Check sheet for the modelled part. Datum: model origin and axes. Units: mm. Face numbers are marked on the shaded views. A direction names the side the tool comes from. Coordinates: 2 decimals unless noted, no trailing zeros. Order: outer loops, then holes, each group sorted by start corner. A loop starts at its lowest first (then second) coordinate and runs counter-clockwise, first axis right, second up.
1. Set-up check for the marked faces 1 and 2: record each of +Z, -Z, +X, -X, +Y, -Y from which the full face is reachable in a straight line by a thin tool's end or side.
2. Cross-section at B-B (z = 38.1). Enter the section's corners in (x, y) (3 decimals).
3. Cross-section at D-D (x = -26). Enter the section's corners in (y, z).
4. Cross-section at C-C (y = 27). Enter the section's corners in (x, z) (3 decimals), then the cut area to 3 significant figures.
5. Thickness scan on line 1 (X direction, y = 22, z = -49.5) (3 decimals); line 2 (Y direction, x = -1.2, z = -38.1); line 3 (Y direction, x = -2.3, z = 38.1). Record the ranges inside material, lowest first.
6. Gauge pin test, flat ends, axial feed: pin 1 Ø12 at (y, z) = (11.5, -4) entering from +X; pin 2 Ø5 at (y, z) = (-4.5, -12) entering from -X; pin 3 Ø8 at (y, z) = (20.06, 38.1) entering from -X (3 decimals); pin 4 Ø6 at (x, z) = (-16, -49.5) entering from +Y. Record the tip position at first contact, or that the pin passes through.
7. Cross-section at A-A (z = 2.5). Enter the section's corners in (x, y) (3 decimals), then the cut area to 3 significant figures.
```python
from build123d import *

# Parameters (mm, degrees)
BOSS_EXTRUDE1_DEPTH               = 63.5
F_1_4_CLEARANCE_HOLE1_D           = 6.7564
F_1_4_CLEARANCE_HOLE1_ON_FACE_2_D = 6.7564


with BuildPart() as part:
    # Sketch1 → Boss-Extrude1 (new body, symmetric)
    with BuildSketch(Plane.XY):
        Polygon((0, 0), (0, 38.1), (-3.175, 38.1), (-3.175, 2.022698078), (-35.872139667, -13.224228548), (-34.530326686, -16.101755772), align=None)
    extrude(amount=BOSS_EXTRUDE1_DEPTH, both=True)

    # 1/4 Clearance Hole1 (through all)
    with Locations(Plane(origin=(-3.175, 20.061349039, -38.1), x_dir=(0, 0, -1), z_dir=(-1, 0, 0))):
        with Locations((0, 0), (-76.2, 0)):
            Hole(F_1_4_CLEARANCE_HOLE1_D / 2)

    # 1/4 Clearance Hole1 on face 2 (through all)
    with Locations(Plane(origin=(-19.523569834, -5.600765235, -38.1), x_dir=(0.906307925, 0.422617965, 0), z_dir=(-0.422617965, 0.906307925, 0))):
        with Locations((0, 0), (0, -76.2)):
            Hole(F_1_4_CLEARANCE_HOLE1_ON_FACE_2_D / 2)


solid = part.part
```
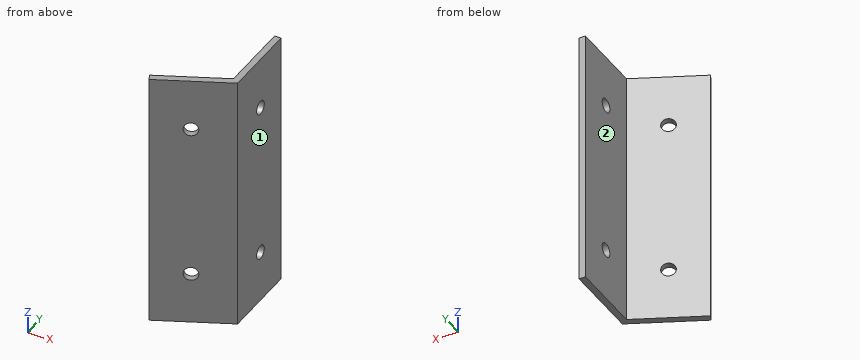
Data:
1. face 1: +Z, -Z, +X, +Y, -Y
1. face 2: +Z, -Z, -X, +Y
2. outline: (-35.872, -13.224) - (-34.53, -16.102) - (-21.243, -9.906) - (-22.585, -7.028) - close; (-16.462, -4.173) - (-15.12, -7.051) - (0, 0) - (0, 16.683) - (-3.175, 16.683) - (-3.175, 2.023) - close; (-3.175, 23.44) - (0, 23.44) - (0, 38.1) - (-3.175, 38.1) - close
3. outline: (-12.12, -63.5) - (-8.62, -63.5) - (-8.62, 63.5) - (-12.12, 63.5) - close
4. outline: (-3.175, -63.5) - (0, -63.5) - (0, 63.5) - (-3.175, 63.5) - close
4. area: 403 mm2
5. line 1: x = -3.175 to 0
5. line 2: y = -0.56 to 16.68, 23.44 to 38.1
5. line 3: y = -1.07 to 16.68, 23.44 to 38.1
6. pin 1: stops at x = 0
6. pin 2: stops at x = -22.52
6. pin 3: stops at x = -3.175
6. pin 4: stops at y = -2.56
7. outline: (-35.872, -13.224) - (-34.53, -16.102) - (0, 0) - (0, 38.1) - (-3.175, 38.1) - (-3.175, 2.023) - close
7. area: 236 mm2
